```python
from build123d import *

# Parameters (mm, degrees)
F1_DEPTH = 3.81
F2_R     = 12.7


with BuildPart() as f1:
    # F0 (on Front) → F1 (new body)
    with BuildSketch(Plane.XZ):
        Polygon((82.55, 25.4), (0, 44.45), (0, -44.45), (82.55, -25.4), align=None)
        with BuildLine():
            ThreePointArc((12.7, -6.604), (6.096, 0), (12.7, 6.604))
            Line((12.7, 6.604), (63.5, 6.604))
            ThreePointArc((63.5, 6.604), (70.104, 0), (63.5, -6.604))
            Line((63.5, -6.604), (12.7, -6.604))
        make_face(mode=Mode.SUBTRACT)
    extrude(amount=F1_DEPTH)

    # F2
    f2_edges = [f1.edges().sort_by_distance(p)[0] for p in [
        (82.55, -1.905, 25.4),
        (82.55, -1.905, -25.4),
    ]]
    fillet(f2_edges, radius=F2_R)


solid = f1.part
```
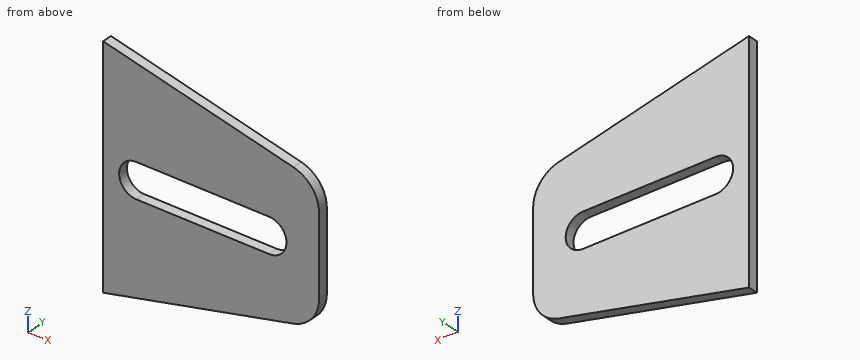
The model under review builds one solid part; all positions refer to its coordinate system, in mm. Round coordinates to 2 decimals unless told otherwise and drop trailing zeros. Write each loop counter-clockwise with the first axis right and the second up, starting at its lowest first coordinate (ties: lowest second). Pieces come first, ordered by that corner, then holes. Notation, with made-up numbers: (-39, 70) - (-10, 70) arc R25 cw to (-10, 92) - close; hole circle Ø10 at (-27, -7). An arc over 180 degrees is marked (long way). One line per question, with ' | ' between items.
Item 1: Add section D-D, the plane z = -25.5. Give the boundary of the cut face in (x, y), then the cut area to 3 significant figures.
Resolved:
outline: (0, -3.81) - (77.41, -3.81) - (77.41, 0) - (0, 0) - close | area: 295 mm2
Item 2: Add section C-C, the plane z = 0. Give the boundary of the cut face in (x, y).
Resolved:
outline: (0, -3.81) - (6.1, -3.81) - (6.1, 0) - (0, 0) - close; (70.1, -3.81) - (82.55, -3.81) - (82.55, 0) - (70.1, 0) - close
Item 3: Add section A-A, the plane y = -2.1. Give the boundary of the cut face in (x, z).
Resolved:
outline: (0, -44.45) - (72.71, -27.67) arc R12.7 ccw to (82.55, -15.3) - (82.55, 15.3) arc R12.7 ccw to (72.71, 27.67) - (0, 44.45) - close; hole (12.7, -6.6) - (63.5, -6.6) arc R6.6 ccw to (63.5, 6.6) - (12.7, 6.6) arc R6.6 ccw to start
Item 4: To check wall thickness, follow probe 1 along Z at (x, y) = (67, -2); probe 2 along X at (y, z) = (-3.4, -2.5); probe 3 along Z at (x, y) = (39, -2.05). State the ranges of each line that lie inside material, in increasing order.
Resolved:
probe 1: z = -28.99 to -5.6, 5.6 to 28.99 | probe 2: x = 0 to 6.59, 69.61 to 82.55 | probe 3: z = -35.45 to -6.6, 6.6 to 35.45
Item 5: Add section B-B, the plane x = 52. Give the boundary of the cut face in (y, z).
Resolved:
outline: (-3.81, -32.45) - (0, -32.45) - (0, -6.6) - (-3.81, -6.6) - close; (-3.81, 6.6) - (0, 6.6) - (0, 32.45) - (-3.81, 32.45) - close
